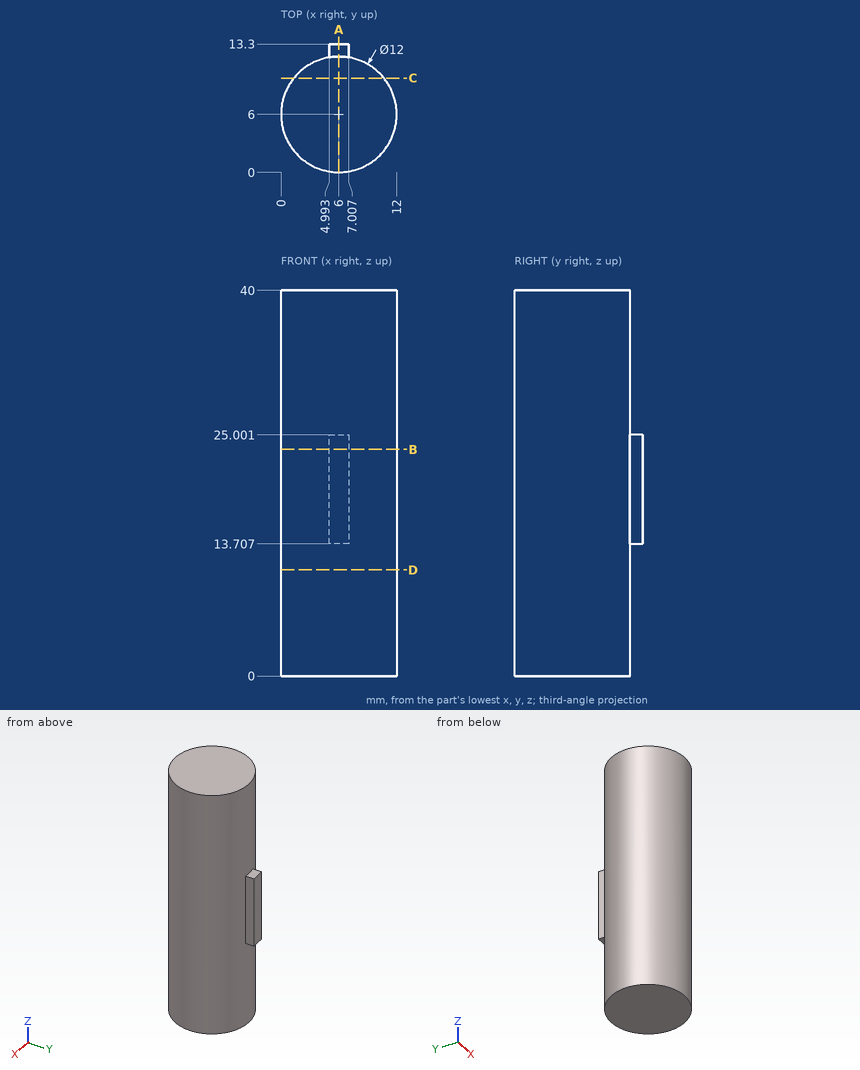
Can you work these out from the drawing? Everything is in mm from the part's minimum corner. Round coordinates to 2 decimals unless told otherwise and drop trailing zeros. Loops run counter-clockwise (first coordinate to the right, second up) from the corner with the lowest first, then second, coordinate; pieces in that order, holes last. Notation, with made-up numbers: (-12.75, 47) -> (6.25, 47) arc R16 ccw to (6.25, 51) -> close; hole circle Ø8 at (1.5, 34). An arc over 180 degrees is marked (long way). Answer in a Markdown table with one row per item.
Item 1: Suppose I cut it at D-D, the plane z = 11. List the corners of the cut face in (x, y) for me, plus the area to 3 significant figures.
Answer block:
| item | result |
|---|---|
| outline | circle Ø12 at (6, 6) |
| area | 113 mm² |
Item 2: Suppose I cut it at C-C, the plane y = 9.75. List the corners of the cut face in (x, z) for me, plus the area to 3 significant figures.
Answer block:
| item | result |
|---|---|
| outline | (1.32, 0) -> (10.68, 0) -> (10.68, 40) -> (1.32, 40) -> close |
| area | 375 mm² |
Item 3: Suppose I cut it at A-A, the plane x = 6. List the corners of the cut face in (y, z) for me.
Answer block:
| item | result |
|---|---|
| outline | (0, 0) -> (12, 0) -> (12, 13.71) -> (13.3, 13.71) -> (13.3, 25) -> (12, 25) -> (12, 40) -> (0, 40) -> close |
Item 4: If I drill on probe 1 along X at (y, z) = (9.5, 16) (1 decimal); probe 2 along Y at (x, z) = (1.5, 6.5), over which ranges is the centre line in solid material (lowest first)?
Answer block:
| item | result |
|---|---|
| probe 1 | 1.1 to 10.9 |
| probe 2 | 2.03 to 9.97 |
Item 5: Suppose I cut it at B-B, the plane z = 23.5. List the corners of the cut face in (x, y) for me (1 decimal), plus the area to 3 significant figures.
Answer block:
| item | result |
|---|---|
| outline | (5, 11.9) arc R6 ccw (long way) to (7, 11.9) -> (7, 13.3) -> (5, 13.3) -> close |
| area | 116 mm² |
Item 6: Will these pins go through, and if not, where does the flat tip stop? P1, Ø0.7, axis at x = 6, y = 12.5, coming from the +Z side; P2, Ø1, axis at y = 10.5, z = 18, coming from the +X side; P3, Ø1.5, axis at x = 8, z = 18, coming from the -Y side.
Answer block:
| item | result |
|---|---|
| P1 | z = 25 |
| P2 | x = 10.47 |
| P3 | y = 0.13 |
